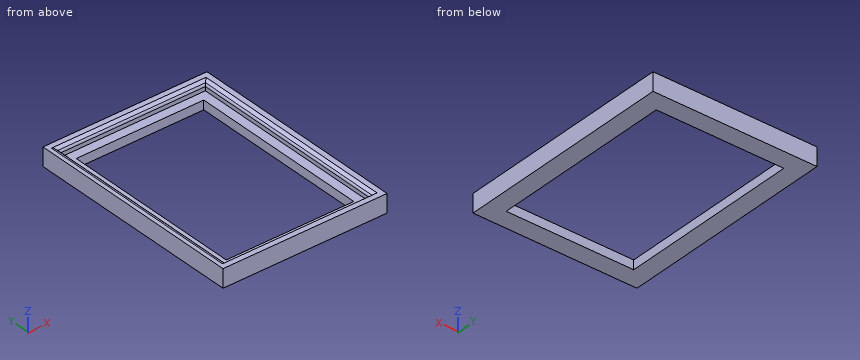
from build123d import *

# Parameters (mm, degrees)
F0_W     = 228.6
F0_H     = 304.8
F0_W_2   = 203.2
F0_H_2   = 279.4
F1_DEPTH = 25.4
F0_W_3   = 177.8
F0_H_3   = 254
F2_DEPTH = 12.7
F3_SIZE  = 5.08
F4_F1_R  = 5.08
F4_F2_R  = 5.08
F4_F3_R  = 5.08
F4_F4_R  = 5.08


with BuildPart() as f1:
    # F0 (on Top) → F1 (new body)
    with BuildSketch(Plane.XY):
        with Locations((114.3, 152.4)):
            Rectangle(F0_W, F0_H)
        with Locations((114.3, 152.4)):
            Rectangle(F0_W_2, F0_H_2, mode=Mode.SUBTRACT)
    extrude(amount=F1_DEPTH)

    # F0 (on Top) → F2 (join)
    with BuildSketch(Plane.XY):
        with Locations((114.3, 152.4)):
            Rectangle(F0_W_2, F0_H_2)
        with Locations((114.3, 152.4)):
            Rectangle(F0_W_3, F0_H_3, mode=Mode.SUBTRACT)
    extrude(amount=F2_DEPTH)

    # F3
    f3_edges = [f1.edges().sort_by_distance(p)[0] for p in [
        (114.3, 292.1, 25.4),
        (215.9, 152.4, 25.4),
        (12.7, 152.4, 25.4),
        (114.3, 12.7, 25.4),
    ]]
    chamfer(f3_edges, length=F3_SIZE)

    # F4: fillet of radius 5.08 on 4 edges, made by hand

    # F4_f1
    f4_f1_edges = [f1.edges().sort_by_distance(p)[0] for p in [
        (7.62, 152.4, 25.4),
    ]]
    fillet(f4_f1_edges, radius=F4_F1_R)

    # F4_f2
    f4_f2_edges = [f1.edges().sort_by_distance(p)[0] for p in [
        (114.3, 292.1, 20.32),
    ]]
    fillet(f4_f2_edges, radius=F4_F2_R)

    # F4_f3
    f4_f3_edges = [f1.edges().sort_by_distance(p)[0] for p in [
        (215.9, 152.6281435083, 20.32),
    ]]
    fillet(f4_f3_edges, radius=F4_F3_R)

    # F4_f4
    f4_f4_edges = [f1.edges().sort_by_distance(p)[0] for p in [
        (114.5281435083, 12.7, 20.32),
    ]]
    fillet(f4_f4_edges, radius=F4_F4_R)


solid = f1.part
Build history of the part. All positions in model axes, mm. Give positions to 0.01 mm unless a question says otherwise; leave off trailing zeros. Loops run counter-clockwise (first coordinate to the right, second up) from the corner with the lowest first, then second, coordinate; pieces in that order, holes last. Notation, with made-up numbers: (82, 57) - (136, 57) arc R27 cw to (136, 74) - close; hole circle Ø2 at (4, 31.5). An arc over 180 degrees is marked (long way). Write item = value, one per line. Start each with the question number.
1) Band-saw the part on C-C on z = 6.75. Give the cut face in (x, y), plus the area to 3 significant figures.
2) Band-saw the part on B-B on x = 188.5. Give the cut face in (y, z), plus the area to 3 significant figures.
3) Probe probe 1 along Y at (x, z) = (171, 5.75); probe 2 along X at (y, z) = (170, 18.5); probe 3 along X at (y, z) = (150, 1). List the from-to ranges inside material, lowest first. Write a range as from..to.
4) Band-saw the part on A-A on y = 216. Give the cut face in (x, z), plus the area to 3 significant figures.
Final values:
q1.outline = (0, 0) - (228.6, 0) - (228.6, 304.8) - (0, 304.8) - close; hole (25.4, 25.4) - (203.2, 25.4) - (203.2, 279.4) - (25.4, 279.4) - close
q1.area = 24,500 mm²
q2.outline = (0, 0) - (25.4, 0) - (25.4, 12.7) - (12.7, 12.7) - (12.7, 18.22) arc R5.08 ccw to (11.21, 21.81) - (7.62, 25.4) - (0, 25.4) - close; (279.4, 0) - (304.8, 0) - (304.8, 25.4) - (297.18, 25.4) - (293.59, 21.81) arc R5.08 ccw to (292.1, 18.22) - (292.1, 12.7) - (279.4, 12.7) - close
q2.area = 941 mm²
q3.probe_1 = 0..25.4, 279.4..304.8
q3.probe_2 = 0..12.7, 215.91..228.6
q3.probe_3 = 0..25.4, 203.2..228.6
q4.outline = (0, 0) - (25.4, 0) - (25.4, 12.7) - (12.7, 12.7) - (12.7, 20.32) - (9.11, 23.91) arc R5.08 ccw to (5.52, 25.4) - (0, 25.4) - close; (203.2, 0) - (228.6, 0) - (228.6, 25.4) - (220.98, 25.4) - (217.39, 21.81) arc R5.08 ccw to (215.9, 18.22) - (215.9, 12.7) - (203.2, 12.7) - close
q4.area = 941 mm²
